from build123d import *

# Parameters (mm, degrees)
SKETCH_1_W          = 75.913642727
SKETCH_1_H          = 62.446702165
EXTRUDE_1_DEPTH     = 2
EXTRUDE_2_DEPTH     = 27
CUT_EXTRUDE_START   = -7
SKETCH_3_W          = 2.124318213
SKETCH_3_H          = 42.832192033
CUT_EXTRUDE_1_DEPTH = 20
SKETCH_4_W          = 2.124318213
SKETCH_4_H          = 7.801964605
EXTRUDE_3_DEPTH     = 10
SKETCH_5_W          = 75.913642727
SKETCH_5_H          = 72.264822367
EXTRUDE_4_DEPTH     = 2
SKETCH_6_W          = 2.124318213
SKETCH_6_H          = 74.38914058
EXTRUDE_5_DEPTH     = 27
SKETCH_7_W          = 21.257465039
SKETCH_7_H          = 58.185991571
EXTRUDE_6_DEPTH     = 2
EXTRUDE_7_DEPTH     = 3
EXTRUDE_START       = 18
EXTRUDE_8_DEPTH     = 3
EXTRUDE_9_DEPTH     = 3
EXTRUDE_10_DEPTH    = 21
CUT_EXTRUDE_START_2 = -8
SKETCH_12_W         = 10.730208879
SKETCH_12_H         = 1.699417316
SKETCH_12_W_2       = 1.944586737
SKETCH_12_H_2       = 11.195277622
SKETCH_12_H_3       = 12.58207638
SKETCH_12_W_3       = 7.811884166
SKETCH_12_H_4       = 1.726665101
CUT_EXTRUDE_2_DEPTH = 10
CUT_EXTRUDE_START_3 = -5.5
SKETCH_13_W         = 2.124318213
SKETCH_13_H         = 31.292512657
CUT_EXTRUDE_3_DEPTH = 10
SKETCH_14_W         = 73.789324514
SKETCH_14_H         = 2.124318213
EXTRUDE_11_DEPTH    = 27
SKETCH_15_W         = 28.654102471
SKETCH_15_H         = 134.711524532
EXTRUDE_12_DEPTH    = 2
SKETCH_16_W         = 28.654102471
SKETCH_16_H         = 2.124318213
SKETCH_16_W_2       = 26.529784258
EXTRUDE_13_DEPTH    = 27
SKETCH_17_W         = 34.092899776
SKETCH_17_H         = 134.711524532
EXTRUDE_14_DEPTH    = 2
SKETCH_18_W         = 2.255075416
SKETCH_18_H         = 46.30769884
EXTRUDE_15_DEPTH    = 27
SKETCH_19_W         = 7.801964605
SKETCH_19_H         = 7.760030918
CUT_EXTRUDE_4_DEPTH = 17
SKETCH_20_W         = 2.124318213
SKETCH_20_H         = 22.381297739
SKETCH_20_W_2       = 34.092899776
SKETCH_20_H_2       = 2.124318213
EXTRUDE_16_DEPTH    = 27
SKETCH_22_W         = 138.660644974
SKETCH_22_H         = 32.329085963
EXTRUDE_17_DEPTH    = 2
SKETCH_23_W         = 136.536326761
SKETCH_23_H         = 2.124318213
EXTRUDE_18_DEPTH    = 27
CUT_EXTRUDE_START_4 = -27
SKETCH_24_W         = 73.789324514
SKETCH_24_H         = 2.124318213
CUT_EXTRUDE_5_DEPTH = 27
SKETCH_25_W         = 3.039057747
SKETCH_25_H         = 29.223543377
EXTRUDE_19_DEPTH    = 27
CUT_EXTRUDE_START_5 = -4.5
SKETCH_26_W         = 88.139659128
SKETCH_26_H         = 19.232592482
CUT_EXTRUDE_6_DEPTH = 14.5
SKETCH_27_W         = 11.249085033
SKETCH_27_H         = 2.124318213
CUT_EXTRUDE_7_DEPTH = 17
SKETCH_28_W         = 3.329603522
SKETCH_28_H         = 47.759206415
SKETCH_28_H_2       = 31.34786159
EXTRUDE_20_DEPTH    = 27
SKETCH_29_W         = 9.233976249
SKETCH_29_H         = 2.124318213
SKETCH_29_W_2       = 3.329603522
SKETCH_29_H_2       = 9.234531485
CUT_EXTRUDE_8_DEPTH = 13.5


with BuildPart() as part:
    # 草图1 → 凸台-拉伸1 (new body)
    with BuildSketch(Plane(origin=(0, 0, 0), x_dir=(1, 0, 0), z_dir=(0, 1, 0))):
        with Locations((37.956821364, -31.223351083)):
            Rectangle(SKETCH_1_W, SKETCH_1_H)
    extrude(amount=EXTRUDE_1_DEPTH)

    # 草图2 → 凸台-拉伸2 (add)
    with BuildSketch(Plane(origin=(0, 2, 0), x_dir=(1, 0, 0), z_dir=(0, 1, 0))):
        Polygon((0, -62.446702165), (75.913642727, -62.446702165), (75.913642727, 0), (0, 0), (0, -52.520419347), (2.124318213, -52.520419347), (2.124318213, -2.124318213), (73.789324514, -2.124318213), (73.789324514, -60.322383952), (68.344319435, -60.322383952), (0, -60.322383952), align=None)
    extrude(amount=EXTRUDE_2_DEPTH)

    # 草图3 → 切除-拉伸1 (cut)
    with BuildSketch(Plane(origin=(0, 29, 0), x_dir=(1, 0, 0), z_dir=(0, 1, 0)).offset(CUT_EXTRUDE_START)):
        with Locations((74.851483621, -29.879654035)):
            Rectangle(SKETCH_3_W, SKETCH_3_H)
    extrude(amount=-CUT_EXTRUDE_1_DEPTH, mode=Mode.SUBTRACT)

    # 草图4 → 凸台-拉伸3 (add)
    with BuildSketch(Plane(origin=(0, 29, 0), x_dir=(1, 0, 0), z_dir=(0, 1, 0))):
        with Locations((1.062159107, -56.421401649)):
            Rectangle(SKETCH_4_W, SKETCH_4_H)
    extrude(amount=-EXTRUDE_3_DEPTH)

    # 草图5 → 凸台-拉伸4 (add)
    with BuildSketch(Plane.XZ):
        with Locations((37.956821364, 98.579113349)):
            Rectangle(SKETCH_5_W, SKETCH_5_H)
    extrude(amount=-EXTRUDE_4_DEPTH)

    # 草图6 → 凸台-拉伸5 (add)
    with BuildSketch(Plane(origin=(0, 2, 0), x_dir=(1, 0, 0), z_dir=(0, 1, 0))):
        with Locations((74.851483621, -97.516954242)):
            Rectangle(SKETCH_6_W, SKETCH_6_H)
    extrude(amount=EXTRUDE_5_DEPTH)

    # 草图7 → 凸台-拉伸6 (add)
    with BuildSketch(Plane.XZ):
        with Locations((86.542375247, 29.092995786)):
            Rectangle(SKETCH_7_W, SKETCH_7_H)
    extrude(amount=-EXTRUDE_6_DEPTH)

    # 草图8 → 凸台-拉伸7 (add)
    with BuildSketch(Plane(origin=(0, 2, 0), x_dir=(1, 0, 0), z_dir=(0, 1, 0))):
        Polygon((75.913642727, -58.185991571), (75.913642727, -56.45932647), (95.226521029, -56.45932647), (95.226521029, -1.699417316), (75.913642727, -1.699417316), (75.913642727, 0), (97.171107766, 0), (97.171107766, -58.185991571), align=None)
    extrude(amount=EXTRUDE_7_DEPTH)

    # 草图9 → 凸台-拉伸8 (add)
    with BuildSketch(Plane(origin=(0, 5, 0), x_dir=(1, 0, 0), z_dir=(0, 1, 0)).offset(EXTRUDE_START)):
        Polygon((75.913642727, -58.185991571), (97.171107766, -58.185991571), (97.171107766, 0), (75.913642727, 0), (75.913642727, -1.699417316), (95.226521029, -1.699417316), (95.226521029, -56.45932647), (75.913642727, -56.45932647), align=None)
    extrude(amount=EXTRUDE_8_DEPTH)

    # 草图10 → 凸台-拉伸9 (add)
    with BuildSketch(Plane(origin=(0, 26, 0), x_dir=(1, 0, 0), z_dir=(0, 1, 0))):
        Polygon((75.913642727, -56.45932647), (75.913642727, -58.185991571), (97.171107766, -58.185991571), (97.171107766, 0), (75.913642727, 0), (75.913642727, -1.699417316), (95.226521029, -1.699417316), (95.226521029, -56.45932647), align=None)
    extrude(amount=EXTRUDE_9_DEPTH)

    # 草图11 → 凸台-拉伸10 (add)
    with BuildSketch(Plane(origin=(0, 5, 0), x_dir=(1, 0, 0), z_dir=(0, 1, 0))):
        Polygon((75.913642727, -56.879985146), (75.913642727, -57.767002905), (96.519280812, -57.767002905), (96.519280812, -0.469783288), (75.913642727, -0.469783288), (75.913642727, -1.183025895), (95.892442802, -1.183025895), (95.892442802, -56.879985146), align=None)
    extrude(amount=EXTRUDE_10_DEPTH)

    # 草图12 → 切除-拉伸2 (cut)
    with BuildSketch(Plane(origin=(0, 29, 0), x_dir=(1, 0, 0), z_dir=(0, 1, 0)).offset(CUT_EXTRUDE_START_2)):
        with Locations((84.386634544, -0.849708658)):
            Rectangle(SKETCH_12_W, SKETCH_12_H)
        with Locations((96.198814398, -12.98486795)):
            Rectangle(SKETCH_12_W_2, SKETCH_12_H_2)
        with Locations((96.198814398, -40.926726277)):
            Rectangle(SKETCH_12_W_2, SKETCH_12_H_3)
        with Locations((87.905733133, -57.32265902)):
            Rectangle(SKETCH_12_W_3, SKETCH_12_H_4)
    extrude(amount=-CUT_EXTRUDE_2_DEPTH, mode=Mode.SUBTRACT)

    # 草图13 → 切除-拉伸3 (cut)
    with BuildSketch(Plane(origin=(0, 29, 0), x_dir=(1, 0, 0), z_dir=(0, 1, 0)).offset(CUT_EXTRUDE_START_3)):
        with Locations((74.851483621, -84.761912061)):
            Rectangle(SKETCH_13_W, SKETCH_13_H)
    extrude(amount=-CUT_EXTRUDE_3_DEPTH, mode=Mode.SUBTRACT)

    # 草图14 → 凸台-拉伸11 (add)
    with BuildSketch(Plane(origin=(0, 2, 0), x_dir=(1, 0, 0), z_dir=(0, 1, 0))):
        with Locations((36.894662257, -106.023590927)):
            Rectangle(SKETCH_14_W, SKETCH_14_H)
    extrude(amount=EXTRUDE_11_DEPTH)

    # 草图15 → 凸台-拉伸12 (add)
    with BuildSketch(Plane.XZ):
        with Locations((-14.327051236, 67.355762266)):
            Rectangle(SKETCH_15_W, SKETCH_15_H)
    extrude(amount=-EXTRUDE_12_DEPTH)

    # 草图16 → 凸台-拉伸13 (add)
    with BuildSketch(Plane(origin=(0, 2, 0), x_dir=(1, 0, 0), z_dir=(0, 1, 0))):
        with Locations((-14.327051236, -1.062159107)):
            Rectangle(SKETCH_16_W, SKETCH_16_H)
        with Locations((-13.264892129, -49.49417616)):
            Rectangle(SKETCH_16_W_2, SKETCH_16_H)
        Polygon((-28.654102471, -62.446702165), (-26.529784258, -62.446702165), (-26.529784258, -50.556335266), (-26.529784258, -48.432017053), (-28.654102471, -48.432017053), align=None)
    extrude(amount=EXTRUDE_13_DEPTH)

    # 草图17 → 凸台-拉伸14 (add)
    with BuildSketch(Plane.XZ):
        with Locations((-45.700552359, 67.355762266)):
            Rectangle(SKETCH_17_W, SKETCH_17_H)
    extrude(amount=-EXTRUDE_14_DEPTH)

    # 草图18 → 凸台-拉伸15 (add)
    with BuildSketch(Plane(origin=(0, 2, 0), x_dir=(1, 0, 0), z_dir=(0, 1, 0))):
        Polygon((-60.491926831, -2.124318213), (-28.654102471, -2.124318213), (-28.654102471, 0), (-62.747002247, 0), (-62.747002247, -2.124318213), align=None)
        with Locations((-61.619464539, -25.278167633)):
            Rectangle(SKETCH_18_W, SKETCH_18_H)
        Polygon((-26.529784258, -48.432017053), (-60.491926831, -48.432017053), (-62.747002247, -48.432017053), (-62.747002247, -50.556335266), (-26.529784258, -50.556335266), align=None)
    extrude(amount=EXTRUDE_15_DEPTH)

    # 草图19 → 切除-拉伸4 (cut)
    with BuildSketch(Plane.XZ.offset(-19)):
        with Locations((-9.25141008, 48.683171807)):
            Rectangle(SKETCH_19_W, SKETCH_19_H)
    extrude(amount=CUT_EXTRUDE_4_DEPTH, mode=Mode.SUBTRACT)

    # 草图20 → 凸台-拉伸16 (add)
    with BuildSketch(Plane(origin=(0, 2, 0), x_dir=(1, 0, 0), z_dir=(0, 1, 0))):
        with Locations((-27.591943365, -73.637351034)):
            Rectangle(SKETCH_20_W, SKETCH_20_H)
        with Locations((-45.700552359, -83.765840798)):
            Rectangle(SKETCH_20_W_2, SKETCH_20_H_2)
    extrude(amount=EXTRUDE_16_DEPTH)

    # 草图22 → 凸台-拉伸17 (add)
    with BuildSketch(Plane.XZ):
        with Locations((6.58332024, 150.876067514)):
            Rectangle(SKETCH_22_W, SKETCH_22_H)
    extrude(amount=-EXTRUDE_17_DEPTH)

    # 草图23 → 凸台-拉伸18 (add)
    with BuildSketch(Plane(origin=(0, 2, 0), x_dir=(1, 0, 0), z_dir=(0, 1, 0))):
        with Locations((5.521161133, -133.649365426)):
            Rectangle(SKETCH_23_W, SKETCH_23_H)
    extrude(amount=EXTRUDE_18_DEPTH)

    # 草图24 → 切除-拉伸5 (cut)
    with BuildSketch(Plane(origin=(0, 29, 0), x_dir=(1, 0, 0), z_dir=(0, 1, 0)).offset(CUT_EXTRUDE_START_4)):
        with Locations((36.894662257, -106.023590927)):
            Rectangle(SKETCH_24_W, SKETCH_24_H)
    extrude(amount=CUT_EXTRUDE_5_DEPTH, mode=Mode.SUBTRACT)

    # 草图25 → 凸台-拉伸19 (add)
    with BuildSketch(Plane(origin=(0, 2, 0), x_dir=(1, 0, 0), z_dir=(0, 1, 0))):
        Polygon((75.913642727, -167.040610495), (75.913642727, -134.711524532), (72.710667325, -134.711524532), (72.710667325, -163.935067909), (72.710667325, -167.040610495), align=None)
        Polygon((72.710667325, -167.040610495), (72.710667325, -163.935067909), (-9.186958654, -163.935067909), (-12.226016401, -163.935067909), (-62.747002247, -163.935067909), (-62.747002247, -167.040610495), align=None)
        with Locations((-10.706487528, -149.32329622)):
            Rectangle(SKETCH_25_W, SKETCH_25_H)
    extrude(amount=EXTRUDE_19_DEPTH)

    # 草图26 → 切除-拉伸6 (cut)
    with BuildSketch(Plane(origin=(0, 29, 0), x_dir=(1, 0, 0), z_dir=(0, 1, 0)).offset(CUT_EXTRUDE_START_5)):
        with Locations((31.843813163, -149.88949865)):
            Rectangle(SKETCH_26_W, SKETCH_26_H)
    extrude(amount=-CUT_EXTRUDE_6_DEPTH, mode=Mode.SUBTRACT)

    # 草图27 → 切除-拉伸7 (cut)
    with BuildSketch(Plane(origin=(0, 29, 0), x_dir=(1, 0, 0), z_dir=(0, 1, 0)).offset(CUT_EXTRUDE_START_4)):
        with Locations((0.435624052, -133.649365426)):
            Rectangle(SKETCH_27_W, SKETCH_27_H)
    extrude(amount=CUT_EXTRUDE_7_DEPTH, mode=Mode.SUBTRACT)

    # 草图28 → 凸台-拉伸20 (add)
    with BuildSketch(Plane(origin=(0, 2, 0), x_dir=(1, 0, 0), z_dir=(0, 1, 0))):
        with Locations((-61.082200486, -108.707603112)):
            Rectangle(SKETCH_28_W, SKETCH_28_H)
        with Locations((-61.082200486, -148.261137114)):
            Rectangle(SKETCH_28_W, SKETCH_28_H_2)
    extrude(amount=EXTRUDE_20_DEPTH)

    # 草图29 → 切除-拉伸8 (cut)
    with BuildSketch(Plane(origin=(0, 29, 0), x_dir=(1, 0, 0), z_dir=(0, 1, 0)).offset(CUT_EXTRUDE_START_4)):
        with Locations((-52.783158211, -133.649365426)):
            Rectangle(SKETCH_29_W, SKETCH_29_H)
        with Locations((-61.082200486, -122.464998081)):
            Rectangle(SKETCH_29_W_2, SKETCH_29_H_2)
    extrude(amount=CUT_EXTRUDE_8_DEPTH, mode=Mode.SUBTRACT)


solid = part.part
CAD build for the part. Positions are in the model's coordinates, mm. A direction names the side the tool comes from. Give positions to 0.01 mm unless a question says otherwise; leave off trailing zeros. Order: outer loops, then holes, each group sorted by start corner. A loop starts at its lowest first (then second) coordinate and runs counter-clockwise, first axis right, second up. Notation, with made-up numbers: (27, 27) -> (61, 27) arc R32 cw to (61, 64) -> close; hole circle Ø6 at (-38.5, 36.25). An arc over 180 degrees is marked (long way). Return JSON: item names as keys, results as strings.
Q1. Mould opens along X. For faces 1 (the face through (-46, 15, 82.704)), 2 (the face through (-62.747, 1, 82)), 3 (the face through (-30, 15, 48.432)) say: pulls with the +X half, pulls with the -X half, needs draft (parallel to the pull), parting line crosses it, or undercut.
Working result:
{"face 1": "needs draft", "face 2": "pulls with the -X half", "face 3": "undercut"}
Q2. Which spindle directions (+Z, -Z, +X, -X, +Y, -Y) get a long thin tool onto all of the face, cutting with end or side? Do faces 4 (the face through (18, 14, 0)), 5 (the face through (-46, 2, 67)), 6 (the face through (95.5, 23, 28.9)), 7 (the face through (73.789, 12, 98)). Say none if no direction does.
Working result:
{"face 4": "-Z, +X, -X, +Y, -Y", "face 5": "-X, +Y", "face 6": "none", "face 7": "+Y"}
Q3. Saw through at C-C (x = -52). Write the cut outline in (y, z), then the cut area to 3 significant figures.
Working result:
{"outline": "(0, 0) -> (29, 0) -> (29, 2.12) -> (2, 2.12) -> (2, 48.43) -> (29, 48.43) -> (29, 50.56) -> (2, 50.56) -> (2, 82.7) -> (29, 82.7) -> (29, 84.83) -> (2, 84.83) -> (2, 163.94) -> (29, 163.94) -> (29, 167.04) -> (0, 167.04) -> close; (15.5, 132.59) -> (29, 132.59) -> (29, 134.71) -> (15.5, 134.71) -> close", "area": "619 mm²"}
Q4. Saw through at A-A (z = 23). Write the cut outline in (x, y), then the cut area to 3 significant figures.
Working result:
{"outline": "(-62.75, 0) -> (97.17, 0) -> (97.17, 5) -> (96.52, 5) -> (96.52, 23) -> (97.17, 23) -> (97.17, 29) -> (95.23, 29) -> (95.23, 23) -> (95.89, 23) -> (95.89, 5) -> (95.23, 5) -> (95.23, 2) -> (2.12, 2) -> (2.12, 29) -> (0, 29) -> (0, 2) -> (-60.49, 2) -> (-60.49, 29) -> (-62.75, 29) -> close; (73.79, 22) -> (75.91, 22) -> (75.91, 29) -> (73.79, 29) -> close", "area": "482 mm²"}
Q5. Drill centre lines: line 1 (Z direction, x = 6, y = 7.75); line 2 (Z direction, x = 13.5, y = 6.5); line 3 (X direction, y = 27.5, z = 148). Where is each one in solid material? Low to high.
Working result:
{"line 1": "0 to 2.12, 60.32 to 62.45, 163.94 to 167.04", "line 2": "0 to 2.12, 60.32 to 62.45, 132.59 to 134.71, 163.94 to 167.04", "line 3": "-62.75 to -59.42, -12.23 to -9.19, 72.71 to 75.91"}
Q6. Saw through at B-B (x = 58). Write the cut outline in (y, z).
Working result:
{"outline": "(0, 0) -> (29, 0) -> (29, 2.12) -> (2, 2.12) -> (2, 60.32) -> (29, 60.32) -> (29, 62.45) -> (2, 62.45) -> (2, 132.59) -> (29, 132.59) -> (29, 134.71) -> (2, 134.71) -> (2, 163.94) -> (29, 163.94) -> (29, 167.04) -> (0, 167.04) -> close"}
Q7. Saw through at D-D (z = 137.5). Write the cut outline in (x, y), then the cut area to 3 significant figures.
Working result:
{"outline": "(-62.75, 0) -> (75.91, 0) -> (75.91, 29) -> (72.71, 29) -> (72.71, 2) -> (-9.19, 2) -> (-9.19, 29) -> (-12.23, 29) -> (-12.23, 2) -> (-59.42, 2) -> (-59.42, 29) -> (-62.75, 29) -> close", "area": "536 mm²"}
Q8. Flat gauge pins, fed straight in: pin 1 (3.5 mm diameter, centred on x = 89.5, y = 3, fed in from +Z); pin 2 (3 mm diameter, centred on x = 60.5, z = 107, fed in from +Y); pin 3 (9 mm diameter, centred on x = 83.5, y = 14, fed in from -Z). Where does each tip first touch, or does it go through?
Working result:
{"pin 1": "z = 58.19", "pin 2": "y = 2", "pin 3": "z = 0.47"}
